For this review, use the dimensioned drawing (mm, ordinates from the lowest corner) and the shaded views. A direction names the side the tool comes from. Coordinates: 2 decimals unless noted, no trailing zeros. Loops run counter-clockwise (first coordinate to the right, second up) from the corner with the lowest first, then second, coordinate; pieces in that order, holes last. Notation, with made-up numbers: (59.5, 86) -> (102.5, 86) arc R26 ccw to (102.5, 121) -> close; hole circle Ø11 at (12.25, 61). An arc over 180 degrees is marked (long way). One line per question, with ' | ' between items. Start each with the question number.
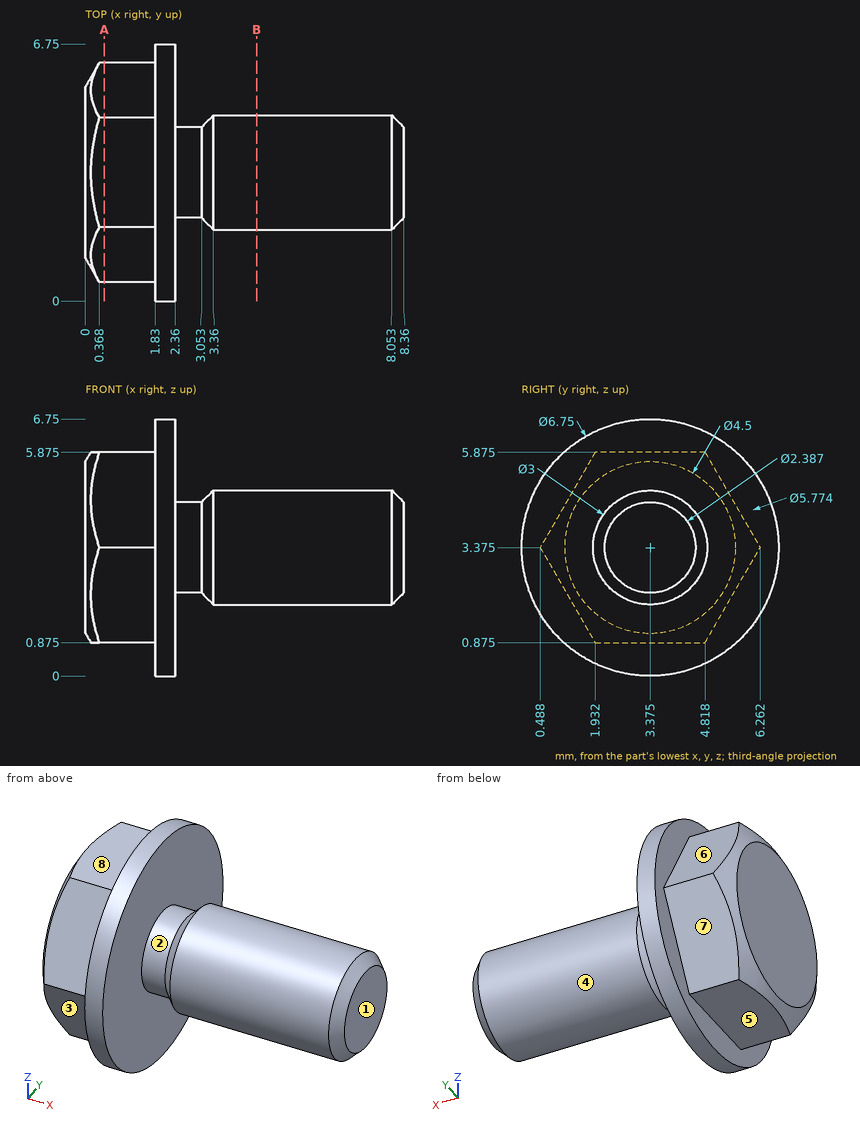
1) Consider section A-A, the plane x = 0.5. Write out the cut boundary in (y, z) (1 decimal).
2) Consider section B-B, the plane x = 4.5. Write out the cut boundary in (y, z) (1 decimal).
3) Insertion check: pin 1 Ø0.8 at (x, y) = (1, 3) entering from +Z (3 decimals); pin 2 Ø4 at (x, z) = (5.5, 0.5) entering from +Y. Each pin has a flat end and moves straight along its axis. Give the tip position at first contact, or say it passes through.
4) Wall thickness on L1, parallel to X at y = 2, z = 2.5; L2, parallel to X at y = 1.75, z = 5.75; L3, parallel to Y at x = 7.75, z = 2.5 (1 decimal): over which ranges is each line inside the solid? List them lowest first.
5) Machinability: for the marked faces 4, 5, 6, 7 and 8, which of the approach directions +Z, -Z, +X, -X, +Y, -Y give a long, thin tool a straight path to every point of the face, cutting with its end or side? Answer none if there is none.
6) Mouldability with a two-part tool opening along X and no side actions: class the marked faces 1, 2 and 3 as +X half, -X half, draft (parallel to the pull), parting line (faces both ways), or undercut.
Filled sheet:
1) outline: (0.5, 3.4) -> (1.9, 0.9) -> (4.8, 0.9) -> (6.3, 3.4) -> (4.8, 5.9) -> (1.9, 5.9) -> close
2) outline: circle Ø3 at (3.4, 3.4)
3) pin 1: z = 5.875 | pin 2: y = 4.59
4) L1: 0 to 2.36 | L2: 1.83 to 2.36 | L3: 2.2 to 4.6
5) face 4: +X | face 5: -Z, -X, +Y, -Y | face 6: +Z, -X, +Y | face 7: -Z, -X, +Y | face 8: +Z, -X, +Y, -Y
6) face 1: +X half | face 2: undercut | face 3: draft
